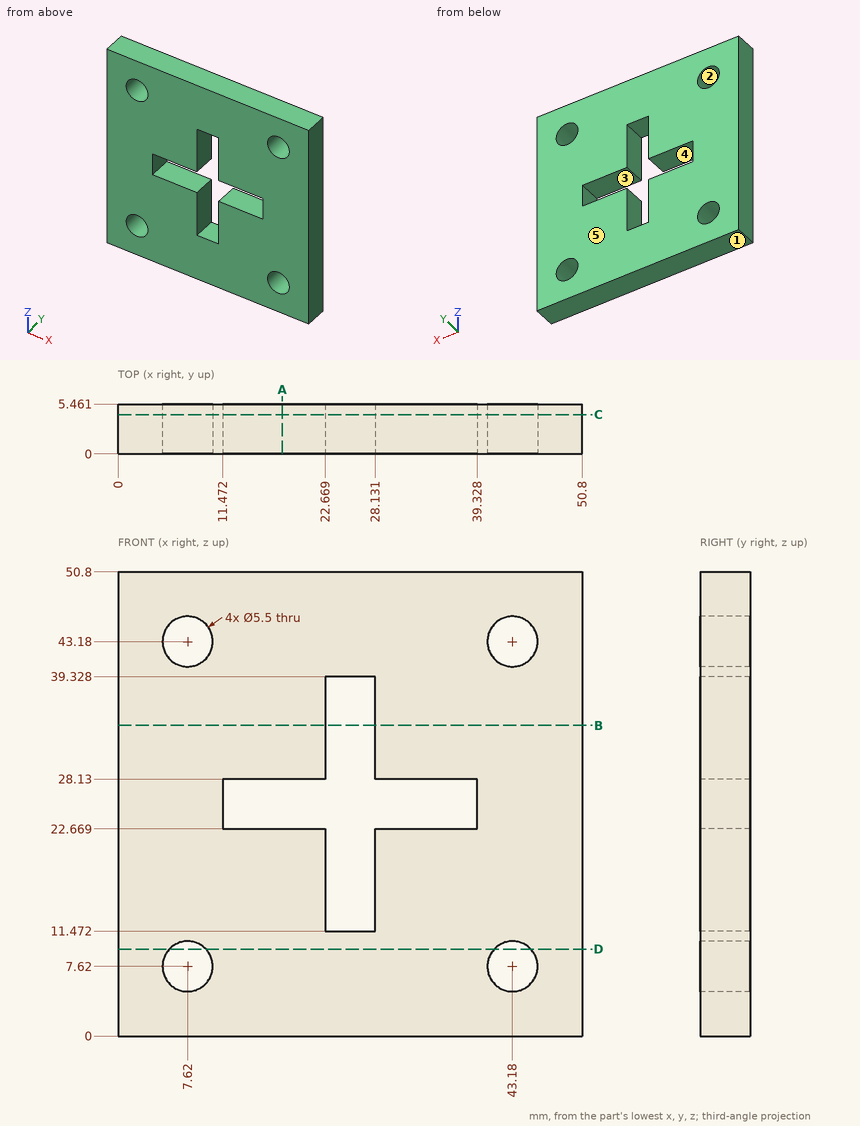
Can you work these out from the drawing? Everything is in mm from the part's minimum corner. A direction names the side the tool comes from. Coordinates: 2 decimals unless noted, no trailing zeros. Order: outer loops, then holes, each group sorted by start corner. A loop starts at its lowest first (then second) coordinate and runs counter-clockwise, first axis right, second up. Notation, with made-up numbers: (71, 56) -> (125, 56) arc R20 cw to (125, 95) -> close; hole circle Ø9 at (15, 35.5). An arc over 180 degrees is marked (long way). Use one line per item in the form item = value.
Q1. Imagine slicing it at C-C, the plane y = 4.3. List the corners of the cut face in (x, z) for me.
From the geometry:
outline = (0, 0) -> (50.8, 0) -> (50.8, 50.8) -> (0, 50.8) -> close; hole circle Ø5.5 at (7.62, 7.62); hole circle Ø5.5 at (7.62, 43.18); hole (11.47, 22.67) -> (22.67, 22.67) -> (22.67, 11.47) -> (28.13, 11.47) -> (28.13, 22.67) -> (39.33, 22.67) -> (39.33, 28.13) -> (28.13, 28.13) -> (28.13, 39.33) -> (22.67, 39.33) -> (22.67, 28.13) -> (11.47, 28.13) -> close; hole circle Ø5.5 at (43.18, 7.62); hole circle Ø5.5 at (43.18, 43.18)
Q2. Imagine slicing it at A-A, the plane x = 18. List the corners of the cut face in (y, z) for me.
From the geometry:
outline = (0, 0) -> (5.46, 0) -> (5.46, 22.67) -> (0, 22.67) -> close; (0, 28.13) -> (5.46, 28.13) -> (5.46, 50.8) -> (0, 50.8) -> close
Q3. I need wall thicknesses on L1, parallel to X at y = 2.9, z = 43.18; L2, parallel to Z at x = 23, y = 1.3. Which ranges of each line are inside material? Lowest first, please.
From the geometry:
L1 = 0 to 4.87, 10.37 to 40.43, 45.93 to 50.8
L2 = 0 to 11.47, 39.33 to 50.8
Q4. Imagine slicing it at D-D, the plane z = 9.5. List the corners of the cut face in (x, y) for me.
From the geometry:
outline = (0, 0) -> (5.61, 0) -> (5.61, 5.46) -> (0, 5.46) -> close; (9.63, 0) -> (41.17, 0) -> (41.17, 5.46) -> (9.63, 5.46) -> close; (45.19, 0) -> (50.8, 0) -> (50.8, 5.46) -> (45.19, 5.46) -> close
Q5. We'd pull the mould along X, two halves only. Please class the marked faces 1, 2 and 3: released by +X, released by -X, zero draft, split by the parting line, or undercut.
From the geometry:
face_1 = zero draft
face_2 = undercut
face_3 = undercut
Q6. Which directions (+Z, -Z, +X, -X, +Y, -Y) give clear straight access to the entire face, cutting with the end or side of a thin tool? Please do the marked faces 4 and 5.
From the geometry:
face_4 = +Y, -Y
face_5 = +Z, -Z, +X, -X, +Y
Q7. Imagine slicing it at B-B, the plane z = 34. List the corners of the cut face in (x, y) for me.
From the geometry:
outline = (0, 0) -> (22.67, 0) -> (22.67, 5.46) -> (0, 5.46) -> close; (28.13, 0) -> (50.8, 0) -> (50.8, 5.46) -> (28.13, 5.46) -> close
